Build history of the part. All positions in model axes, mm. A direction names the side the tool comes from. Give positions to 0.01 mm unless a question says otherwise; leave off trailing zeros. Write each loop counter-clockwise with the first axis right and the second up, starting at its lowest first coordinate (ties: lowest second). Pieces come first, ordered by that corner, then holes. Notation, with made-up numbers: (-39, 65) -> (0, 65) arc R22 ccw to (0, 98) -> close; hole circle Ø10 at (31.5, -23). An arc over 180 degrees is marked (long way). Write item = value, one per line. Start each with the question number.
Q1. Saw through at A-A, the plane y = 26. List the corners of the cut face in (x, z), then the cut area to 3 significant figures.
Q2. Tool access for faces 5 (the face through (48.6, -31.01, 3.98)), 6 (the face through (-45.473, 27, 87)), 7 (the face through (1.9, -49.27, 97.5)): list every direction of +Z, -Z, +X, -X, +Y, -Y with a clear straight run to the whole face (end or side of a thin tool).
Q3. Mould opens along Y. For faces 1 (the face through (-5, 19.069, 99)), 2 (the face through (1.898, 45.577, 97.496)), 3 (the face through (-44.898, -2.476, 2.504)), 4 (the face through (41, -31, 2)) say: pulls with the +Y half, pulls with the -Y half, needs draft (parallel to the pull), parting line crosses it, or undercut.
Q4. Drop flat-ended pins along their axis: P1, Ø5.5, axis at x = 43, y = -29, coming from the -Z side; P2, Ø8, axis at x = -10, y = 27.5, coming from the +Z side; P3, Ø1, axis at x = -46.5, y = 26, coming from the +Z side. Give the stop position or say it passes through.
Q5. Wall check: line 1 (X direction, y = 31.5, z = 38); line 2 (Z direction, x = -12, y = 20.5); line 3 (Z direction, x = 37, y = -31). Give the ranges that are in metal, low to high.
from build123d import *

# Parameters (mm, degrees)
F0_W      = 100
F0_H      = 100
F1_DEPTH  = 100
F2_SIZE   = 5.08
F3_W      = 89.84
F3_H      = 16.256
F4_DEPTH  = 2
F5_W      = 16.256
F5_H      = 7.1842048969
F6_DEPTH  = 2
F7_W      = 16.256
F7_H      = 14.2303462458
F8_DEPTH  = 2
F9_W      = 16.256
F9_H      = 7.1842048969
F10_DEPTH = 2
F11_W     = 16.256
F11_H     = 64.0321317446
F12_DEPTH = 2
F13_W     = 16.256
F13_H     = 64.03213
F14_DEPTH = 2
F15_W     = 16.256
F15_H     = 7.1842048969
F16_DEPTH = 2
F17_W     = 11.9421218839
F17_H     = 16.256
F18_DEPTH = 2


with BuildPart() as f1:
    # F0 (on Top) → F1 (new body)
    with BuildSketch(Plane.XY):
        with Locations((2.5266306475, -1.8473280194)):
            Rectangle(F0_W, F0_H)
    extrude(amount=F1_DEPTH)

    # F2
    f2_edges = [f1.edges().sort_by_distance(p)[0] for p in [
        (2.526631, -51.847328, 100),
        (-47.473369, -1.847328, 100),
        (-47.473369, -51.847328, 50),
        (52.526631, -51.847328, 50),
        (2.526631, -51.847328, 0),
        (52.526631, -1.847328, 0),
        (2.526631, 48.152672, 0),
        (52.526631, 48.152672, 50),
        (-47.473369, 48.152672, 50),
        (-47.473369, -1.847328, 0),
        (2.526631, 48.152672, 100),
        (52.526631, -1.847328, 100),
    ]]
    chamfer(f2_edges, length=F2_SIZE)

    # F3 (on face) → F4 (cut)
    with BuildSketch(Plane.XY.offset(100)):
        with Locations((2.5266306475, 27.1967347203)):
            Rectangle(F3_W, F3_H)
    extrude(amount=-F4_DEPTH, mode=Mode.SUBTRACT)

    # F5 (on face) → F6 (cut)
    with BuildSketch(Plane(origin=(-71.1966846763, 0, 71.1966846763), x_dir=(0, -1, 0), z_dir=(-0.7071067812, 0, 0.7071067812))):
        with Locations((-27.1967347203, 37.1419367237)):
            Rectangle(F5_W, F5_H)
    extrude(amount=-F6_DEPTH, mode=Mode.SUBTRACT)

    # F7 (on face) → F8 (cut)
    with BuildSketch(Plane(origin=(-47.4733693525, 0, 0), x_dir=(0, -1, 0), z_dir=(-1, 0, 0))):
        with Locations((-27.1967347203, 87.8048268771)):
            Rectangle(F7_W, F7_H)
    extrude(amount=-F8_DEPTH, mode=Mode.SUBTRACT)

    # F9 (on face) → F10 (cut)
    with BuildSketch(Plane(origin=(73.7233153237, 0, 73.7233153237), x_dir=(0, 1, 0), z_dir=(0.7071067812, 0, 0.7071067812))):
        with Locations((27.1967347203, 33.5687413949)):
            Rectangle(F9_W, F9_H)
    extrude(amount=-F10_DEPTH, mode=Mode.SUBTRACT)

    # F11 (on face) → F12 (cut)
    with BuildSketch(Plane.YZ.offset(52.5266306475)):
        with Locations((27.1967347203, 62.9039341277)):
            Rectangle(F11_W, F11_H)
    extrude(amount=-F12_DEPTH, mode=Mode.SUBTRACT)

    # F13 (on face) → F14 (cut)
    with BuildSketch(Plane.YZ.offset(52.5266306475)):
        with Locations((-30.8923280194, 37.096065)):
            Rectangle(F13_W, F13_H)
    extrude(amount=-F14_DEPTH, mode=Mode.SUBTRACT)

    # F15 (on face) → F16 (cut)
    with BuildSketch(Plane(origin=(23.7233153237, 0, -23.7233153237), x_dir=(0, 1, 0), z_dir=(0.7071067812, 0, -0.7071067812))):
        with Locations((-30.8923280194, 37.1419367237)):
            Rectangle(F15_W, F15_H)
    extrude(amount=-F16_DEPTH, mode=Mode.SUBTRACT)

    # F17 (on face) → F18 (cut)
    with BuildSketch(Plane(origin=(0, 0, 0), x_dir=(1, 0, 0), z_dir=(0, 0, -1))):
        with Locations((41.4755697055, 30.8923280194)):
            Rectangle(F17_W, F17_H)
    extrude(amount=-F18_DEPTH, mode=Mode.SUBTRACT)


solid = f1.part
Report:
q1.outline = (-47.47, 5.08) -> (-42.39, 0) -> (47.45, 0) -> (52.53, 5.08) -> (52.53, 30.89) -> (50.53, 30.89) -> (50.53, 94.09) -> (46.62, 98) -> (-41.56, 98) -> (-45.47, 94.09) -> (-45.47, 80.69) -> (-47.47, 80.69) -> close
q1.area = 9,590 mm2
q2.face_5 = -Z, +X
q2.face_6 = +Z, -X
q2.face_7 = +Z, +X, -X, -Y
q3.face_1 = undercut
q3.face_2 = pulls with the +Y half
q3.face_3 = needs draft
q3.face_4 = undercut
q4.P1 = 2
q4.P2 = 98
q4.P3 = 80.69
q5.line_1 = -47.47 to 50.53
q5.line_2 = 0 to 98
q5.line_3 = 2 to 100
